from build123d import *

# Parameters (mm, degrees)
F0_R     = 11
F1_DEPTH = 1


with BuildPart() as f1:
    # F0 (on Front) → F1 (new body)
    with BuildSketch(Plane.XZ):
        with BuildLine():
            ThreePointArc((-20.2, 55), (-20.815670936, 58.7123282218), (-22.5967618828, 62.0271655581))
            ThreePointArc((-22.5967618828, 62.0271655581), (-42.0061632577, 60.1022542964), (-31.7688713732, 43.5002062308))
            ThreePointArc((-31.7688713732, 43.5002062308), (-23.5926582899, 46.8439586565), (-20.2, 55))
        make_face()
        with Locations((-31.7, 55)):
            Circle(F0_R, mode=Mode.SUBTRACT)
        with BuildLine():
            Line((-20, 20), (-12.7, 20))
            Line((-12.7, 20), (-12.7, 45.7048399691))
            ThreePointArc((-12.7, 45.7048399691), (-14.7065803005, 53.9638063884), (-20.2789473684, 60.3814084389))
            Line((-20.2789473684, 60.3814084389), (-22.5967618828, 62.0271655581))
            ThreePointArc((-22.5967618828, 62.0271655581), (-20.815670936, 58.7123282218), (-20.2, 55))
            ThreePointArc((-20.2, 55), (-23.5926582899, 46.8439586565), (-31.7688713732, 43.5002062308))
            Line((-31.7688713732, 43.5002062308), (-45.3524999934, -6.6727046639))
            ThreePointArc((-45.3524999934, -6.6727046639), (-45.6127443207, -7.9678442227), (-45.7, -9.2859868679))
            Line((-45.7, -9.2859868679), (-45.7, -10))
            ThreePointArc((-45.7, -10), (-42.7710678119, -17.0710678119), (-35.7, -20))
            Line((-35.7, -20), (-20, -20))
            Line((-20, -20), (-20, 20))
        make_face()
        with BuildLine():
            ThreePointArc((-32.7, -3), (-31.8213203436, -0.8786796564), (-29.7, 0))
            Line((-29.7, 0), (-28.7, 0))
            ThreePointArc((-28.7, 0), (-26.5786796564, -0.8786796564), (-25.7, -3))
            Line((-25.7, -3), (-25.7, -15))
            ThreePointArc((-25.7, -15), (-26.5786796564, -17.1213203436), (-28.7, -18))
            Line((-28.7, -18), (-29.7, -18))
            ThreePointArc((-29.7, -18), (-31.8213203436, -17.1213203436), (-32.7, -15))
            Line((-32.7, -15), (-32.7, -3))
        make_face(mode=Mode.SUBTRACT)
        with BuildLine():
            Line((-12.7, 20), (-12.7, -1.15e-08))
            Line((-12.7, -1.15e-08), (-12.7, -20))
            Line((-12.7, -20), (15, -20))
            ThreePointArc((15, -20), (18.5355339059, -18.5355339059), (20, -15))
            Line((20, -15), (20, 15))
            ThreePointArc((20, 15), (18.5355339059, 18.5355339059), (15, 20))
            Line((15, 20), (-12.7, 20))
        make_face()
        with BuildLine():
            ThreePointArc((-12.7, -1.15e-08), (-5.7e-09, 12.7), (12.7, 0))
            ThreePointArc((12.7, 0), (5.7e-09, -12.7), (-12.7, -1.15e-08))
        make_face(mode=Mode.SUBTRACT)
        Polygon((-12.7, -20), (-12.7, -1.15e-08), (-12.7, 20), (-20, 20), (-20, -20), align=None)
    extrude(amount=F1_DEPTH)


solid = f1.part
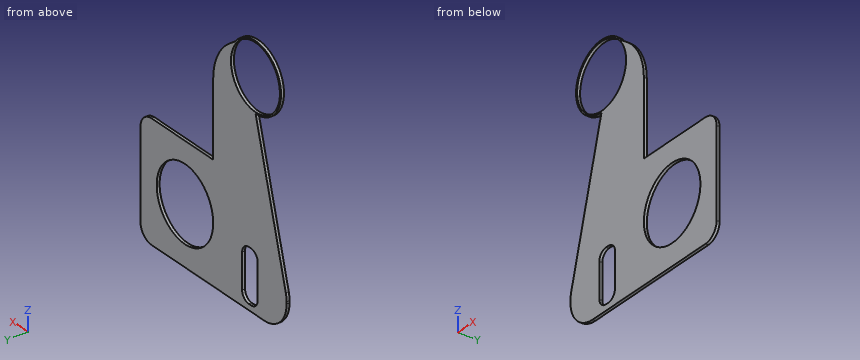
Verification items for the finished model (mm, model axes). Give positions to 0.01 mm unless a question says otherwise; leave off trailing zeros. Write each loop counter-clockwise with the first axis right and the second up, starting at its lowest first coordinate (ties: lowest second). Pieces come first, ordered by that corner, then holes.
(1) Gauge pin test, flat ends, axial feed: pin 1 (17.5 mm diameter, centred on x = -31.7, z = 55, fed in from -Y); pin 2 (4 mm diameter, centred on x = -24, z = -3, fed in from +Y); pin 3 (0.5 mm diameter, centred on x = -29, y = -0.5, fed in from +Z); pin 4 (0.5 mm diameter, centred on x = 0.5, y = -0.5, fed in from +Z). Record the tip position at first contact, or that the pin passes through.
(2) Cross-section at A-A (z = 8). Enter the section's corners in (x, y).
(3) Cross-section at C-C (y = -0.75). Enter the section's corners in (x, z).
(4) Cross-section at D-D (x = -34). Enter the section's corners in (y, z), plus the area to 3 significant figures.
(5) Cross-section at B-B (x = 0). Enter the section's corners in (y, z).
(6) Material ranges on line 1 (Z direction, x = 0, y = -0.3); line 2 (Z direction, x = -31.7, y = -0.3); line 3 (Z direction, x = 15, y = -0.15), recorded low to high.
Worked out:
1. pin 1: passes through
1. pin 2: stops at y = 0
1. pin 3: stops at z = 66.24
1. pin 4: stops at z = 20
2. outline: (-41.38, -1) - (-9.86, -1) - (-9.86, 0) - (-41.38, 0) - close; (9.86, -1) - (20, -1) - (20, 0) - (9.86, 0) - close
3. outline: (-45.7, -10) arc R10 ccw to (-35.7, -20) - (15, -20) arc R5 ccw to (20, -15) - (20, 15) arc R5 ccw to (15, 20) - (-12.7, 20) - (-12.7, 45.7) arc R18 ccw to (-20.28, 60.38) - (-22.6, 62.03) arc R11.5 ccw (long way) to (-31.77, 43.5) - (-45.35, -6.67) arc R10 ccw to (-45.7, -9.29) - close; hole circle Ø22 at (-31.7, 55); hole (-32.7, -15) arc R3 ccw to (-29.7, -18) - (-28.7, -18) arc R3 ccw to (-25.7, -15) - (-25.7, -3) arc R3 ccw to (-28.7, 0) - (-29.7, 0) arc R3 ccw to (-32.7, -3) - close; hole circle Ø25.4 at (0, 0)
4. outline: (-1, -20) - (0, -20) - (0, 35.26) - (-1, 35.26) - close; (-1, 43.73) - (0, 43.73) - (0, 44.24) - (-1, 44.24) - close; (-1, 65.76) - (0, 65.76) - (0, 66.27) - (-1, 66.27) - close
4. area: 56.3 mm2
5. outline: (-1, -20) - (0, -20) - (0, -12.7) - (-1, -12.7) - close; (-1, 12.7) - (0, 12.7) - (0, 20) - (-1, 20) - close
6. line 1: z = -20 to -12.7, 12.7 to 20
6. line 2: z = -20 to -17.24, -0.76 to 44, 66 to 66.5
6. line 3: z = -20 to 20
